```python
from build123d import *

# Parameters (mm, degrees)
F0_W      = 41.12726
F0_H      = 110.894836
F1_DEPTH  = 19.05
F3_DEPTH  = 19.05
F5_DEPTH  = 19.05
F6_W      = 27.651456
F6_H      = 74.505314
F7_DEPTH  = 33.02
F9_DEPTH  = 37.084
F11_DEPTH = 37.084
F12_R     = 6.963256
F13_DEPTH = 112.828874
F14_W     = 41.989248
F14_H     = 25.538178
F15_DEPTH = 34.56532
F16_W     = 40.965122
F16_H     = 20.482562
F17_DEPTH = 34.821354
F18_R     = 10.243282
F19_DEPTH = 19.051
F20_R     = 10.356495
F21_DEPTH = 19.051


with BuildPart() as f1:
    # F0 (on Top) → F1 (new body)
    with BuildSketch(Plane.XY):
        Rectangle(F0_W, F0_H)
    extrude(amount=F1_DEPTH)

    # F2 (on Top) → F3 (join)
    with BuildSketch(Plane.XY):
        with BuildLine():
            Line((-20.738592, 55.430926), (20.994626, 55.430926))
            ThreePointArc((20.994626, 55.430926), (0.128017, 75.575216), (-20.738592, 55.430926))
        make_face()
    extrude(amount=F3_DEPTH)

    # F4 (on Top) → F5 (join)
    with BuildSketch(Plane.XY):
        with BuildLine():
            ThreePointArc((-20.56363, -55.447418), (0, -75.683733), (20.56363, -55.447418))
            Line((20.56363, -55.447418), (-20.56363, -55.447418))
        make_face()
    extrude(amount=F5_DEPTH)

    # F6 (on face) → F7 (join)
    with BuildSketch(Plane.XY.offset(19.05)):
        Rectangle(F6_W, F6_H)
    extrude(amount=F7_DEPTH)

    # F8 (on Front) → F9 (join)
    with BuildSketch(Plane.XZ):
        with BuildLine():
            Line((-13.825728, 52.07), (13.825728, 52.07))
            ThreePointArc((13.825728, 52.07), (0, 64.904116), (-13.825728, 52.07))
        make_face()
    extrude(amount=F9_DEPTH)

    # F10 (on Front) → F11 (join)
    with BuildSketch(Plane.XZ):
        with BuildLine():
            Line((-13.825728, 52.07), (13.825728, 52.07))
            ThreePointArc((13.825728, 52.07), (0, 65.062803), (-13.825728, 52.07))
        make_face()
    extrude(amount=-F11_DEPTH)

    # F12 (on face) → F13 (cut, through all)
    with BuildSketch(Plane.XZ.offset(37.252657)):
        with Locations((0, 52.07)):
            Circle(F12_R)
    extrude(amount=-F13_DEPTH, mode=Mode.SUBTRACT)

    # F14 (on face) → F15 (cut, through all)
    with BuildSketch(Plane.YZ.offset(13.825728)):
        with Locations((0, 52.07)):
            Rectangle(F14_W, F14_H)
        with BuildLine():
            Line((20.994624, 39.300911), (-20.994624, 39.300911))
            ThreePointArc((-20.994624, 39.300911), (0, 26.893632), (20.994624, 39.300911))
        make_face()
    extrude(amount=-F15_DEPTH, mode=Mode.SUBTRACT)

    # F16 (on face) → F17 (cut, through all)
    with BuildSketch(Plane(origin=(-13.825728, 0, 0), x_dir=(0, -1, 0), z_dir=(-1, 0, 0))):
        with Locations((0, 56.711089)):
            Rectangle(F16_W, F16_H)
    extrude(amount=-F17_DEPTH, mode=Mode.SUBTRACT)

    # F18 (on face) → F19 (cut, through all)
    with BuildSketch(Plane.XY.offset(19.05)):
        with Locations((0.128017, 54.695657)):
            Circle(F18_R)
    extrude(amount=-F19_DEPTH, mode=Mode.SUBTRACT)

    # F20 (on face) → F21 (cut, through all)
    with BuildSketch(Plane.XY.offset(19.05)):
        with Locations((0, -55.117455)):
            Circle(F20_R)
    extrude(amount=-F21_DEPTH, mode=Mode.SUBTRACT)


solid = f1.part
```
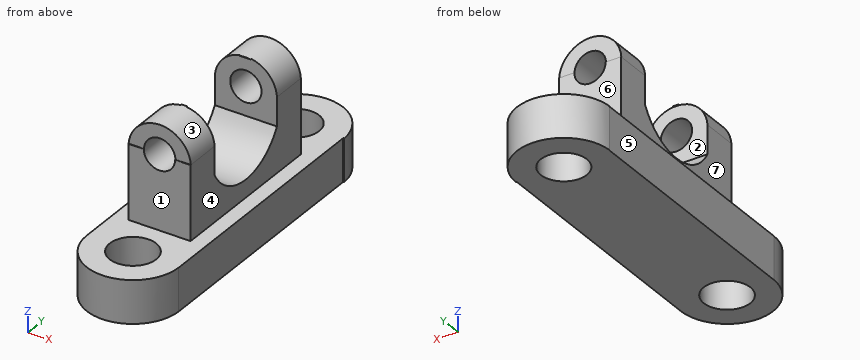
The listing builds one solid part. Answer for the finished solid, in the listing's coordinates (mm). Face numbers are marked on the shaded views. A direction names the side the tool comes from. Give positions to 0.01 mm unless a question says otherwise; leave off trailing zeros. Loops run counter-clockwise (first coordinate to the right, second up) from the corner with the lowest first, then second, coordinate; pieces in that order, holes last. Notation, with made-up numbers: (19.25, -6.5) - (38.25, -6.5) arc R15 ccw to (38.25, 8.5) - close; hole circle Ø9 at (74.5, 62). An arc over 180 degrees is marked (long way). Answer as CSV lines item,"result". Start each with the question number.
Item 1: For the marked faces 4, 5, 6 and 7, determine the directions among +Z, -Z, +X, -X, +Y, -Y from which every point of the face is accessible in a straight line to the end or side of a thin tool.
Item 2: A cutting plane is placed at B-B on z = 4. Determine the outline of the cut face in (x, y), then the cut area to 3 significant figures.
Item 3: Each of these flat-tipped pins is pushed along its axis until it touches: pin 1 (6.5 mm diameter, centred on x = 5.5, z = 61, fed in from -Y); pin 2 (12 mm diameter, centred on x = -10, z = 31, fed in from +Y); pin 3 (21 mm diameter, centred on x = 6.5, y = 32.5, fed in from +Z); pin 4 (9.5 mm diameter, centred on y = 20, z = 7, fed in from -X). Where does it stop, or does it pass through?
Item 4: A cutting plane is placed at A-A on y = -32. Determine the outline of the cut face in (x, z).
Item 5: The mould has two halves that part along Y. Classify the marked faces 1, 2 and 3: +Y half, -Y half, draft (parallel to the pull), parting line (faces both ways), or undercut.
Item 6: A cutting plane is placed at C-C on x = -16.5. Determine the outline of the cut face in (y, z).
Item 7: Find the intervals of material crossed by line 1 (Z direction, x = 0, y = 29); line 2 (Y direction, x = -7, z = 40.5); line 3 (Z direction, x = 16, y = 7.5), in increasing order. Write a range as from..to.
Found:
1,face 4,"+Z, +X, +Y, -Y"
1,face 5,"+Z, -Z, -X, -Y"
1,face 6,"+Z, +X, -X, +Y"
1,face 7,"+Z, -X, +Y, -Y"
2,outline,"(-20.74, 55.43) - (-20.56, 55.43) - (-20.56, -55.45) arc R20.57 ccw to (20.56, -55.45) - (20.56, 55.43) - (20.99, 55.43) arc R20.88 ccw to start; hole circle Ø20.71 at (0, -55.12); hole circle Ø20.49 at (0.13, 54.7)"
2,area,"5,200 mm^2"
3,pin 1,"stops at y = -37.08"
3,pin 2,"stops at y = 37.25"
3,pin 3,"stops at z = 65.06"
3,pin 4,"stops at x = -20.56"
4,outline,"(-20.56, 0) - (20.56, 0) - (20.56, 19.05) - (13.83, 19.05) - (13.83, 52.07) arc R13.86 ccw to (-13.83, 52.07) - (-13.83, 19.05) - (-20.56, 19.05) - close; hole circle Ø13.93 at (0, 52.07)"
5,face 1,"-Y half"
5,face 2,"undercut"
5,face 3,"draft"
6,outline,"(-67.39, 0) - (67.32, 0) - (67.32, 19.05) - (-67.39, 19.05) - close"
7,line 1,"z = 0..45.11, 59.03..65.06"
7,line 2,"y = -37.25..-20.99, 20.99..37.25"
7,line 3,"z = 0..19.05"
